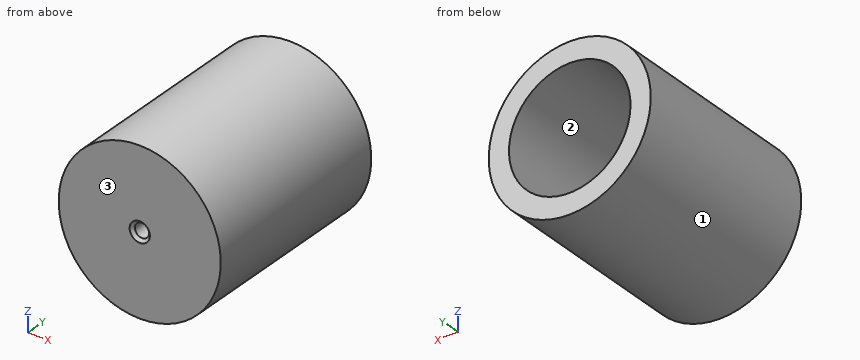
from build123d import *

# Parameters (mm, degrees)
SKETCH2_R           = 10.16
BOSS_EXTRUDE1_DEPTH = 25.4
SKETCH3_R           = 7.62
CUT_EXTRUDE1_DEPTH  = 20.32
SKETCH4_R           = 0.889
CUT_EXTRUDE2_DEPTH  = 3.048
CHAMFER1_SIZE       = 0.381
CHAMFER2_SIZE       = 0.2159
CHAMFER2_SIZE2      = 0.805749769


with BuildPart() as part:
    # Sketch2 → Boss-Extrude1 (new body)
    with BuildSketch(Plane(origin=(0, 0, 0), x_dir=(1, 0, 0), z_dir=(0, 1, 0))):
        with Locations(Location((0, 0, 0), (0, 0, 270))):
            Circle(SKETCH2_R)
    extrude(amount=BOSS_EXTRUDE1_DEPTH)

    # Sketch3 → Cut-Extrude1 (cut)
    with BuildSketch(Plane(origin=(0, 25.4, 0), x_dir=(1, 0, 0), z_dir=(0, 1, 0))):
        with Locations(Location((0, 0, 0), (0, 0, 270))):
            Circle(SKETCH3_R)
    extrude(amount=-CUT_EXTRUDE1_DEPTH, mode=Mode.SUBTRACT)

    # Sketch4 → Cut-Extrude2 (cut)
    with BuildSketch(Plane.XZ):
        with Locations(Location((0, 0, 0), (0, 0, 270))):
            Circle(SKETCH4_R)
    extrude(amount=-CUT_EXTRUDE2_DEPTH, mode=Mode.SUBTRACT)

    # Chamfer1
    chamfer1_edges = [part.edges().sort_by_distance(p)[0] for p in [
        (0, 0, 0.889),
    ]]
    chamfer(chamfer1_edges, length=CHAMFER1_SIZE)

    # Chamfer2
    chamfer2_edges = [part.edges().sort_by_distance(p)[0] for p in [
        (0, 3.048, 0.889),
    ]]
    chamfer2_side = [part.faces().sort_by_distance(p)[0] for p in [
        (0, 1.7145, 0.889),
    ]]
    chamfer(chamfer2_edges, length=CHAMFER2_SIZE, length2=CHAMFER2_SIZE2, reference=chamfer2_side[0])


solid = part.part
CAD build for the part. Positions are in the model's coordinates, mm. Face numbers are marked on the shaded views. Round coordinates to 2 decimals unless told otherwise and drop trailing zeros. Write each loop counter-clockwise with the first axis right and the second up, starting at its lowest first coordinate (ties: lowest second). Pieces come first, ordered by that corner, then holes.
(1) Slice it at D-D, the plane y = 3.75. Write the cut outline in (x, z), and give its area (3 significant figures).
(2) Slice it at A-A, the plane z = 6.5. Write the cut outline in (x, y), and give its area (3 significant figures).
(3) Drop flat-ended pins along their axis: P1, Ø3, axis at y = 16, z = -2.5, coming from the +X side; P2, Ø6, axis at y = 22.5, z = 4.5, coming from the +X side; P3, Ø5, axis at x = -4.5, y = 3, coming from the +Z side. Give the stop position or say it passes through.
(4) Mould opens along Z. For the marked faces 1, 2 and 3 say: pulls with the +Z half, pulls with the -Z half, needs draft (parallel to the pull), parting line crosses it, or undercut.
(5) Slice it at C-C, the plane y = 7.5. Write the cut outline in (x, z), and give its area (3 significant figures).
(6) Slice it at B-B, the plane x = 5.75. Write the cut outline in (y, z), and give its area (3 significant figures).
(7) Probe line 1 along X through (y, z) = (2, 0); line 2 along Y through (x, z) = (1.5, -2); line 3 along Z through (x, y) = (-1.5, 10). List the from-to ranges inside material, lowest first.
From the geometry:
1. outline: circle Ø20.32 at (0, 0)
1. area: 324 mm2
2. outline: (-7.81, 0) - (7.81, 0) - (7.81, 25.4) - (3.98, 25.4) - (3.98, 5.08) - (-3.98, 5.08) - (-3.98, 25.4) - (-7.81, 25.4) - close
2. area: 235 mm2
3. P1: stops at x = 10.11
3. P2: stops at x = 10.05
3. P3: stops at z = 9.96
4. face 1: parting line crosses it
4. face 2: undercut
4. face 3: needs draft
5. outline: circle Ø20.32 at (0, 0); hole circle Ø15.24 at (0, 0)
5. area: 142 mm2
6. outline: (0, -8.38) - (25.4, -8.38) - (25.4, -5) - (5.08, -5) - (5.08, 5) - (25.4, 5) - (25.4, 8.38) - (0, 8.38) - close
6. area: 222 mm2
7. line 1: x = -10.16 to -0.89, 0.89 to 10.16
7. line 2: y = 0 to 5.08
7. line 3: z = -10.05 to -7.47, 7.47 to 10.05
